The model under review builds one solid part; all positions refer to its coordinate system, in mm. A direction names the side the tool comes from. Coordinates: 2 decimals unless noted, no trailing zeros. Loops run counter-clockwise (first coordinate to the right, second up) from the corner with the lowest first, then second, coordinate; pieces in that order, holes last. Notation, with made-up numbers: M -31.75,67 L 11.25,67 A33 cw 11.25,104 Z; hole C 41.25,-34 d1. An arc over 180 degrees is marked long. Use one line per item in the form item = value.
```python
from build123d import *

# Parameters (mm, degrees)
F0_W     = 45.08
F0_H     = 20.08
F0_W_2   = 40
F0_H_2   = 15
F1_DEPTH = 19.05
F2_R     = 1.27
F4_DEPTH = 9


with BuildPart() as f1:
    # F0 (on Top) → F1 (new body)
    with BuildSketch(Plane.XY):
        Rectangle(F0_W, F0_H)
        Rectangle(F0_W_2, F0_H_2, mode=Mode.SUBTRACT)
    extrude(amount=F1_DEPTH)

    # F2
    f2_edges = [f1.edges().sort_by_distance(p)[0] for p in [
        (-20, 7.5, 9.525),
        (-20, -7.5, 9.525),
        (20, 7.5, 9.525),
        (20, -7.5, 9.525),
        (-22.54, -10.04, 9.525),
        (-22.54, 10.04, 9.525),
        (22.54, -10.04, 9.525),
        (22.54, 10.04, 9.525),
    ]]
    fillet(f2_edges, radius=F2_R)

    # F3 (on face) → F4 (join)
    with BuildSketch(Plane.XY.offset(19.05)):
        with BuildLine():
            Line((21.27, 10.04), (-21.27, 10.04))
            ThreePointArc((-21.27, 10.04), (-22.168026, 9.668026), (-22.54, 8.77))
            Line((-22.54, 8.77), (-22.54, -8.77))
            ThreePointArc((-22.54, -8.77), (-22.168026, -9.668026), (-21.27, -10.04))
            Line((-21.27, -10.04), (21.27, -10.04))
            ThreePointArc((21.27, -10.04), (22.168026, -9.668026), (22.54, -8.77))
            Line((22.54, -8.77), (22.54, 8.77))
            ThreePointArc((22.54, 8.77), (22.168026, 9.668026), (21.27, 10.04))
        make_face()
    extrude(amount=F4_DEPTH)


solid = f1.part
```
1. Add section C-C (y = 5.75). State the section outline as (x, z) points.
Response values:
outline = M -22.54,0 L -20,0 L -20,19.05 L 20,19.05 L 20,0 L 22.54,0 L 22.54,28.05 L -22.54,28.05 Z
2. Wall thickness on line 1 along Y through (x, z) = (7.5, 14); line 2 along X through (y, z) = (5, 3.5); line 3 along Z through (x, y) = (-6, -5): over which ranges is each line inside the solid? List them lowest first. Write a range as from..to.
Response values:
line_1 = -10.04..-7.5, 7.5..10.04
line_2 = -22.54..-20, 20..22.54
line_3 = 19.05..28.05
3. Machinability: for faces 4 (the face through (0, -8, 0)), 5 (the face through (0, -7.5, 9)), which of the approach directions +Z, -Z, +X, -X, +Y, -Y give a long, thin tool a straight path to every point of the face, cutting with its end or side? Answer none if there is none.
Response values:
face_4 = -Z, +X, -X, +Y, -Y
face_5 = -Z
4. The part is to be moulded in two halves that separate along X. For faces 1 (the face through (0, 10.04, 14)), 2 (the face through (-22.54, 0, 14)), 3 (the face through (19.638, 7.118, 9.658)), say which applies: pulls with the +X half, pulls with the -X half, needs draft (parallel to the pull), parting line crosses it, or undercut.
Response values:
face_1 = needs draft
face_2 = pulls with the -X half
face_3 = undercut
5. Add section A-A (x = 2.5). State the section outline as (y, z) points.
Response values:
outline = M -10.04,0 L -7.5,0 L -7.5,19.05 L 7.5,19.05 L 7.5,0 L 10.04,0 L 10.04,28.05 L -10.04,28.05 Z
6. Add section B-B (z = 16.25). State the section outline as (x, y) points, then the cut area to 3 significant figures.
Response values:
outline = M -22.54,-8.77 A1.27 ccw -21.27,-10.04 L 21.27,-10.04 A1.27 ccw 22.54,-8.77 L 22.54,8.77 A1.27 ccw 21.27,10.04 L -21.27,10.04 A1.27 ccw -22.54,8.77 Z; hole M -20,-6.23 A1.27 ccw -18.73,-7.5 L 18.73,-7.5 A1.27 ccw 20,-6.23 L 20,6.23 A1.27 ccw 18.73,7.5 L -18.73,7.5 A1.27 ccw -20,6.23 Z
area = 305 mm^2
